Read the model definition and answer for the solid it produces. Units are mm, in the model's axes. A direction names the side the tool comes from. Coordinates: 2 decimals unless noted, no trailing zeros. Order: outer loops, then holes, each group sorted by start corner. A loop starts at its lowest first (then second) coordinate and runs counter-clockwise, first axis right, second up. Notation, with made-up numbers: (14.25, 57.5) - (56.25, 57.5) arc R26 cw to (56.25, 85.5) - close; hole circle Ø9 at (70, -38). An arc over 180 degrees is marked (long way). Write item = value, one per line.
Autodesk Inventor part; units mm, degrees
ref_plane "YZ Plane" through (0, 0, 0) normal (1, 0, 0) x (0, 1, 0)
ref_plane "XZ Plane" through (0, 0, 0) normal (0, 1, 0) x (-1, 0, 0)
ref_plane "XY Plane" through (0, 0, 0) normal (0, 0, 1) x (1, 0, 0)
sketch "Sketch1" plane through (0, 0, 0) normal (0, 0, 1) x (1, 0, 0)
  circle A0 centre (0, 0) radius 265 construction
  line L0 (0, 265) -> (0, 295) construction
  line L1 (0, 265) -> (0, 235) construction
  circle A1 centre (0, 0) radius 235
  circle A2 centre (0, 0) radius 295
  line L2 (-235, 0) -> (-235, 80) construction
  line L3 (-235, 80) -> (-295, 80) construction
  line L4 (-295, 80) -> (-295, 0) construction
  line L5 (235, 0) -> (235, 80) construction
  line L6 (235, 80) -> (295, 80) construction
  line L7 (295, 80) -> (295, 0) construction
  line L8 (-235, 0) -> (-295, 0)
  line L9 (-295, 0) -> (-355, 0)
  line L10 (-355, 0) -> (-355, -50)
  line L11 (-355, -50) -> (-290.7318, -50)
  line L12 (235, 0) -> (295, 0)
  line L13 (295, 0) -> (355, 0)
  line L14 (355, 0) -> (355, -50)
  line L15 (355, -50) -> (290.7318, -50)
  dimension "d13" = 530
  dimension "d26" = 80
  dimension "d36" = 60
  dimension "d40" = 60
  dimension "d41" = 50
extrude "Extrusion1" add sketch "Sketch1" against normal blind 30 contours L12 A2 L8 A1 | L13 L14 L15 A2 | A2 L11 L10 L9 picked at (3.5144, -274.7637)
sketch "Sketch4" plane through (0, 0, 0) normal (0, 0, 1) x (1, 0, 0)
  line L0 (0, 0) -> (51.6989, -259.9081) construction
  line L1 (0, 0) -> (0, -276.8337) construction
  dimension "d27" = 265
  dimension "d35" = 11.25
sketch "Sketch7" plane through (0, 0, 0) normal (0, 0, 1) x (1, 0, 0)
  line L0 (-355, -50) -> (-355, 0) construction
  line L1 (-355, -25) -> (355, -25) construction
  line L2 (355, 0) -> (355, -50) construction
  point P0 (0, 0)
  point P1 (-330, -25)
  dimension "d42" = 25
fillet "Fillet1" [suppressed]
hole "Hole1" [suppressed]
hole "Hole2" at (51.6989, -259.9081, 0) direction (0, 0, -1) diameter 13 end through all counterbore diameter 35 counterbore depth 15
pattern_circular "Circular Pattern4" count 9 over 180 about axis through (0, 0, -10) along (0, 0, -1) of "Hole2" both ways yes
mirror "Mirror1" [suppressed]
sketch "Sketch9" plane through (-355, 0, 0) normal (0, 1, 0) x (1, 0, 0)
  circle A0 centre (25, 15) radius 7
  line L0 (0, 0) -> (0, 30)
  point P0 (355, 0)
  point P1 (0, 15)
  dimension "d70" = 25
  dimension "d71" = 14
extrude "Extrusion8" cut sketch "Sketch9" against normal through all
mirror "Mirror2" about plane through (0, 0, 0) normal (1, 0, 0) of "Extrusion8"
equation "\"d13\" = Шпил_пласт_КОРМА_диам_центров"
equation "\"d40\" = d36"
equation "\"d27\" = 0.5 * Шпил_пласт_КОРМА_диам_центров"
equation "\"BendReliefDepth\" = 0.5 * Thickness"
properties part number "Постель 201 зад"
1) Determine the mould class of faces 4 (the face through (-28, -245, -30)), 5 (the face through (264.889, -55.875, -22.605)), 6 (the face through (355, -25, -15)) for opening direction X: pulls with the +X half, pulls with the -X half, needs draft (parallel to the pull), parting line crosses it, or undercut.
Returned:
face_4 = needs draft
face_5 = undercut
face_6 = pulls with the +X half
2) The part is cut by section B-B (y = -20). Determine the outline of the cut face in (x, z), and give its area (3 significant figures).
Returned:
outline = (-355, -30) - (-234.15, -30) - (-234.15, 0) - (-355, 0) - close; (234.15, -30) - (355, -30) - (355, 0) - (234.15, 0) - close; hole circle Ø14 at (-330, -15); hole circle Ø14 at (330, -15)
area = 6,940 mm^2
3) The part is cut by section C-C (x = 0). Determine the outline of the cut face in (y, z), and give its area (3 significant figures).
Returned:
outline = (-295, -30) - (-235, -30) - (-235, 0) - (-295, 0) - close
area = 1,800 mm^2
4) Flat-ended cylindrical pins translate along their axes: pin 1 Ø18 at (x, z) = (330, -15) entering from -Y; pin 2 Ø15 at (x, y) = (220.34, -147.23) entering from +Z; pin 3 Ø12 at (y, z) = (-152.5, -3.5) entering from +X. Find the tip coordinate at first contact, or state that the pin passes through.
Returned:
pin_1 = -50
pin_2 = -15
pin_3 = 256.05
5) Straight lines are drawn through the part: line 1 along X through (y, z) = (-156, -14); line 2 along X through (y, z) = (-248, -7.5); line 3 along X through (y, z) = (-56.5, -14.5). For each, find the intervals that lie inside material, in ascending order. Write a range as from..to.
Returned:
line_1 = -250.38..-235.48, -205.2..-175.75, 175.75..205.2, 235.48..250.38
line_2 = -159.75..-64.52, -38.88..38.88, 64.52..159.75
line_3 = -289.54..-276.74, -243.08..-228.11, 228.11..243.08, 276.74..289.54
6) For faces 1 (the face through (55.654, -254.75, -22.605)), 2 (the face through (-323, -50, -18)), 3 (the face through (-260, -59, -15)), determine the directions among +Z, -Z, +X, -X, +Y, -Y from which every point of the face is accessible in a straight line to the end or side of a thin tool.
Returned:
face_1 = +Z, -Z
face_2 = +Z, -Z, -X, -Y
face_3 = +Z
7) The part is cut by section A-A (x = 330). Determine the outline of the cut face in (y, z).
Returned:
outline = (-50, -30) - (0, -30) - (0, -22) - (-50, -22) - close; (-50, -8) - (0, -8) - (0, 0) - (-50, 0) - close
